from build123d import *

# Parameters (mm, degrees)
F0_R     = 63.5
F0_R_2   = 2.0955
F0_R_3   = 4.064
F1_DEPTH = 12.7
F3_DEPTH = 12.7
F2_R     = 3.2385
F2_R_2   = 2.0955
F4_DEPTH = 9.525


with BuildPart() as f1:
    # F0 (on Top) → F1 (new body)
    with BuildSketch(Plane.XY):
        with Locations((-27.8360728791, 11.0515514389)):
            Circle(F0_R)
        with Locations((-27.8360728791, 3.0505514389)):
            Circle(F0_R_2, mode=Mode.SUBTRACT)
        with Locations((-35.8370728791, 11.0515514389)):
            Circle(F0_R_2, mode=Mode.SUBTRACT)
        with Locations((-27.8360728791, 11.0515514389)):
            Circle(F0_R_3, mode=Mode.SUBTRACT)
        with Locations((-19.8350728791, 11.0515514389)):
            Circle(F0_R_2, mode=Mode.SUBTRACT)
        with Locations((-27.8360728791, 19.0525514389)):
            Circle(F0_R_2, mode=Mode.SUBTRACT)
    extrude(amount=F1_DEPTH)

    # F2 (on face) → F3 (cut)
    with BuildSketch(Plane.XY.offset(12.7)):
        with BuildLine():
            ThreePointArc((-48.5403226608, 31.0707388843), (-62.0442946523, 42.5994874775), (-70.1548226491, 58.3946968551))
            ThreePointArc((-70.1548226491, 58.3946968551), (-82.8286860194, 42.8015514389), (-89.9958143896, 24.029091088))
            ThreePointArc((-89.9958143896, 24.029091088), (-72.2614978121, 24.9027724934), (-55.5253226608, 18.9723639934))
            ThreePointArc((-55.5253226608, 18.9723639934), (-48.2007234403, 22.8090879223), (-48.5403226608, 31.0707388843))
        make_face()
        with BuildLine():
            ThreePointArc((-20.8510728791, 38.9915514389), (-17.6188697193, 56.450708532), (-7.9950811385, 71.3722365042))
            ThreePointArc((-7.9950811385, 71.3722365042), (-27.8360728791, 74.5515514389), (-47.6770646196, 71.3722365042))
            ThreePointArc((-47.6770646196, 71.3722365042), (-38.0532760389, 56.450708532), (-34.8210728791, 38.9915514389))
            ThreePointArc((-34.8210728791, 38.9915514389), (-27.8360728791, 34.5666244058), (-20.8510728791, 38.9915514389))
        make_face()
        with BuildLine():
            ThreePointArc((34.3236686315, 24.029091088), (27.1565402612, 42.8015514389), (14.4826768909, 58.3946968551))
            ThreePointArc((14.4826768909, 58.3946968551), (6.3721488941, 42.5994874775), (-7.1318230973, 31.0707388843))
            ThreePointArc((-7.1318230973, 31.0707388843), (-7.4714223178, 22.8090879223), (-0.1468230973, 18.9723639934))
            ThreePointArc((-0.1468230973, 18.9723639934), (16.5893520539, 24.9027724934), (34.3236686315, 24.029091088))
        make_face()
        with BuildLine():
            ThreePointArc((14.4826768909, -36.2915939774), (27.1565402612, -20.6984485611), (34.3236686315, -1.9259882102))
            ThreePointArc((34.3236686315, -1.9259882102), (16.5893520539, -2.7996696157), (-0.1468230973, 3.1307388843))
            ThreePointArc((-0.1468230973, 3.1307388843), (-7.4714223178, -0.7059850446), (-7.1318230973, -8.9676360066))
            ThreePointArc((-7.1318230973, -8.9676360066), (6.3721488941, -20.4963845997), (14.4826768909, -36.2915939774))
        make_face()
        with BuildLine():
            ThreePointArc((-47.6770646196, -49.2691336265), (-27.8360728791, -52.4484485611), (-7.9950811385, -49.2691336265))
            ThreePointArc((-7.9950811385, -49.2691336265), (-17.6188697193, -34.3476056543), (-20.8510728791, -16.8884485611))
            ThreePointArc((-20.8510728791, -16.8884485611), (-27.8360728791, -12.4635215281), (-34.8210728791, -16.8884485611))
            ThreePointArc((-34.8210728791, -16.8884485611), (-38.0532760389, -34.3476056543), (-47.6770646196, -49.2691336265))
        make_face()
        with BuildLine():
            ThreePointArc((-55.5253226608, 3.1307388843), (-72.2614978121, -2.7996696157), (-89.9958143896, -1.9259882102))
            ThreePointArc((-89.9958143896, -1.9259882102), (-82.8286860194, -20.6984485611), (-70.1548226491, -36.2915939774))
            ThreePointArc((-70.1548226491, -36.2915939774), (-62.0442946523, -20.4963845997), (-48.5403226608, -8.9676360066))
            ThreePointArc((-48.5403226608, -8.9676360066), (-48.2007234403, -0.7059850446), (-55.5253226608, 3.1307388843))
        make_face()
    extrude(amount=-F3_DEPTH, mode=Mode.SUBTRACT)

    # F2 (on face) → F4 (cut)
    with BuildSketch(Plane.XY.offset(12.7)):
        with Locations((-27.8360728791, 19.0525514389)):
            Circle(F2_R)
        with Locations((-27.8360728791, 19.0525514389)):
            Circle(F2_R_2, mode=Mode.SUBTRACT)
        with Locations((-19.8350728791, 11.0515514389)):
            Circle(F2_R)
        with Locations((-19.8350728791, 11.0515514389)):
            Circle(F2_R_2, mode=Mode.SUBTRACT)
        with Locations((-27.8360728791, 3.0505514389)):
            Circle(F2_R)
        with Locations((-27.8360728791, 3.0505514389)):
            Circle(F2_R_2, mode=Mode.SUBTRACT)
        with Locations((-35.8370728791, 11.0515514389)):
            Circle(F2_R)
        with Locations((-35.8370728791, 11.0515514389)):
            Circle(F2_R_2, mode=Mode.SUBTRACT)
    extrude(amount=-F4_DEPTH, mode=Mode.SUBTRACT)


solid = f1.part
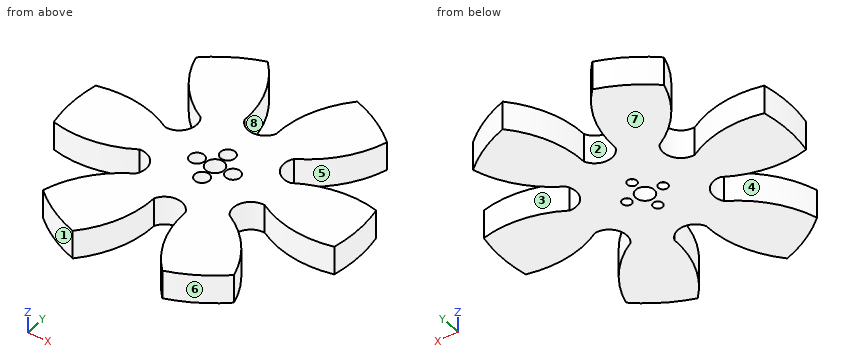
Design review of the part built by this model. Coordinates are the model's own, in mm. Face numbers are marked on the shaded views. A direction names the side the tool comes from. Give positions to 0.01 mm unless a question says otherwise; leave off trailing zeros. Write each loop counter-clockwise with the first axis right and the second up, starting at its lowest first coordinate (ties: lowest second). Pieces come first, ordered by that corner, then holes. Notation, with made-up numbers: M 74.25,-35 L 118.25,-35 A26 cw 118.25,-3 Z; hole C 60.25,-16.5 d4. An arc over 180 degrees is marked long. Answer as a JSON object with one key per item and string values. Group by question number.
1) We need section A-A (y = 44.5). Give the boundary of the cut face in (x, z), and give its area (3 significant figures).
2) We need section D-D (y = -41). Give the boundary of the cut face in (x, z), and give its area (3 significant figures).
3) Clearance check with flat-ended pins moving along their axes: pin 1 Ø8 at (x, y) = (-62, 37.5) entering from +Z; pin 2 Ø1 at (y, z) = (-33.5, 2.5) entering from -X; pin 3 Ø5 at (x, y) = (-27.84, 3.05) entering from +Z (3 decimals); pin 4 Ø6 at (x, z) = (4.5, 10) entering from +Y. State where each tip first meets the part, or that it passes through.
4) We need section B-B (z = 9). Count the separate pieces of the cut face and the enclosed holes in it, and give its area (3 significant figures).
5) For line 1 along X through (y, z) = (11, 3.75); line 2 along Y through (x, z) = (3.5, 5.75); line 3 along X through (y, z) = (10.5, 11.25), list the stretches that pass through material, from the lowest coordinate up.
6) Mouldability with a two-part tool opening along X and no side actions: class the marked faces 6, 7 and 8 as released by +X, released by -X, zero draft, split by the parting line, or undercut.
7) We need section C-C (x = -28). Give the boundary of the cut face in (y, z) (3 decimals), and give its area (3 significant figures).
8) Tool access review of the marked faces 1, 2, 3, 4 and 5: name each direction out of +Z, -Z, +X, -X, +Y, -Y from which nothing blocks a thin tool from reaching the whole face with its end or side.
Answer key:
{
 "1": {"outline": "M -63.47,0 L -35.09,0 L -35.09,12.7 L -63.47,12.7 Z; M -20.58,0 L 7.8,0 L 7.8,12.7 L -20.58,12.7 Z", "area": "721 mm²"},
 "2": {"outline": "M -64.21,0 L -41.34,0 L -41.34,12.7 L -64.21,12.7 Z; M -14.33,0 L 8.54,0 L 8.54,12.7 L -14.33,12.7 Z", "area": "581 mm²"},
 "3": {"pin 1": "stops at z = 12.7", "pin 2": "stops at x = -69.43", "pin 3": "stops at z = 3.175", "pin 4": "stops at y = 67.37"},
 "4": {"separate pieces": "1", "enclosed holes": "5", "area": "7,460 mm²"},
 "5": {"line 1": "x = -91.34 to -39.08, -32.6 to -31.9, -23.77 to -23.07, -16.6 to 35.66", "line 2": "y = -44.18 to -17.2, 1.18 to 20.92, 39.3 to 66.28", "line 3": "x = -91.33 to -39.03, -32.65 to -31.86, -23.81 to -23.03, -16.64 to 35.66"},
 "6": {"face 6": "released by +X", "face 7": "zero draft", "face 8": "undercut"},
 "7": {"outline": "M -12.465,0 L 0.961,0 L 0.961,3.175 L -0.184,3.175 L -0.184,12.7 L -12.465,12.7 Z; M 5.14,0 L 6.991,0 L 6.991,12.7 L 6.285,12.7 L 6.285,3.175 L 5.14,3.175 Z; M 15.112,0 L 16.963,0 L 16.963,3.175 L 15.818,3.175 L 15.818,12.7 L 15.112,12.7 Z; M 21.142,0 L 34.568,0 L 34.568,12.7 L 22.287,12.7 L 22.287,3.175 L 21.142,3.175 Z", "area": "344 mm²"},
 "8": {"face 1": "+Z, -Z, -X, -Y", "face 2": "+Z, -Z, +Y", "face 3": "+Z, -Z", "face 4": "+Z, -Z, -X", "face 5": "+Z, -Z, +X"}
}
